Check sheet for the modelled part. Datum: model origin and axes. Units: mm. A direction names the side the tool comes from. Coordinates: 2 decimals unless noted, no trailing zeros. Write each loop counter-clockwise with the first axis right and the second up, starting at its lowest first coordinate (ties: lowest second). Pieces come first, ordered by that corner, then holes. Notation, with made-up numbers: (19.25, 49) - (30.25, 49) arc R15 ccw to (30.25, 76) - close; hole circle Ø11 at (-18, -28). An arc over 180 degrees is marked (long way). Use one line per item in the form item = value. Start each with the question number.
1. Tool access check on faces 1 (the face through (6, -2, -7)), 2 (the face through (3.436, 13.438, 8.76)), 3 (the face through (8.864, 13.438, 8.76)). Record the directions out of +Z, -Z, +X, -X, +Y, -Y that give a thin tool (end or side, any length) a straight path to the whole face; none if there is none.
2. Go/stop test with flat-tipped pins: pin 1 Ø6 at (x, z) = (8, -16) entering from -Y; pin 2 Ø1 at (x, z) = (3, -0.5) entering from +Y; pin 3 Ø1.4 at (x, y) = (4, 24.5) entering from +Z. Record where each tip stops, or that it passes through.
3. Cross-section at C-C on z = 7. Record the boundary of the cut face in (x, y).
4. Cross-section at D-D on y = 16.5. Record the boundary of the cut face in (x, z), then the cut area to 3 significant figures.
5. Cross-section at B-B on y = 1.5. Record the boundary of the cut face in (x, z).
6. Cross-section at A-A on y = 12.3. Record the boundary of the cut face in (x, z).
7. Draft check along Z on faces 4 (the face through (6.2, 24.9, -4)), 5 (the face through (3, 27.3, -5)), 6 (the face through (6.1, 15.2, 2.2)). Enter one of: +Z half, -Z half, draft (parallel to the pull), parting line (faces both ways), or undercut.
8. Scan lines: line 1 along X through (y, z) = (26.2, -4.95); line 2 along Z through (x, y) = (10, 3.5); line 3 along Z through (x, y) = (8.75, -1.5). Record each from-to range of solid material in increasing order.
Autodesk Inventor part; units mm, degrees
ref_plane "YZ Plane" through (0, 0, 0) normal (1, 0, 0) x (0, 1, 0)
ref_plane "XZ Plane" through (0, 0, 0) normal (0, 1, 0) x (-1, 0, 0)
ref_plane "XY Plane" through (0, 0, 0) normal (0, 0, 1) x (1, 0, 0)
sketch "Sketch1" plane through (0, 0, 0) normal (0, 0, 1) x (1, 0, 0)
  line L0 (0, 0) -> (12.3, 0)
  line L1 (12.3, 0) -> (12.3, 22.6)
  line L2 (12.3, 22.6) -> (0, 22.6)
  line L3 (0, 22.6) -> (0, 0)
  line L4 (6.15, 22.6) -> (6.15, 0) construction
  arc A0 (3.3318, 11.6163) -> (8.9682, 11.6163) centre (6.15, 6.15) ccw
  arc A1 (8.9682, 11.6163) -> (3.3318, 11.6163) centre (6.15, 12.3) ccw
  dimension "d0" = 12.3
  dimension "d1" = 22.6
  dimension "d2" = 6.15
  dimension "d3" = 6.15
  dimension "d4" = 5.8
extrude "Extrusion1" add sketch "Sketch1" against normal blind 22.3
sketch "Sketch2" plane through (0, 0, 0) normal (0, 0, 1) x (1, 0, 0)
  line L0 (0, 0) -> (12.3, 0)
  line L1 (12.3, 0) -> (12.3, 22.6)
  line L2 (12.3, 22.6) -> (0, 22.6)
  line L3 (0, 22.6) -> (0, 0)
  line L4 (6.15, 22.6) -> (6.15, 0) construction
  arc A0 (3.3318, 11.6163) -> (8.9682, 11.6163) centre (6.15, 6.15) ccw
  arc A1 (8.9682, 11.6163) -> (3.3318, 11.6163) centre (6.15, 12.3) ccw
  dimension "d7" = 12.3
  dimension "d8" = 22.6
  dimension "d9" = 6.15
  dimension "d10" = 6.15
  dimension "d11" = 5.8
extrude "Extrusion2" add sketch "Sketch2" along normal blind 4.5 contours A0 A1
sketch "Sketch3" plane through (0, 22.6, 0) normal (0, 1, 0) x (1, 0, 0)
  line L0 (12.3, 0) -> (0, 0) construction
  line L1 (12.3, 0) -> (12.3, 22.3) construction
  line L2 (0, 0) -> (0, 22.3) construction
  line L3 (12.3, 4) -> (0, 4)
  line L4 (0, 4) -> (0, 6.5)
  line L5 (0, 6.5) -> (12.3, 6.5)
  line L6 (12.3, 6.5) -> (12.3, 4)
  dimension "d14" = 4
  dimension "d15" = 2.5
extrude "Extrusion3" add sketch "Sketch3" along normal blind 4.7
sketch "Sketch4" plane through (0, 0, -22.3) normal (0, -1, 0) x (1, 0, 0)
  line L0 (12.3, 15.3) -> (0, 15.3)
  line L1 (0, 15.3) -> (0, 17.8)
  line L2 (0, 17.8) -> (12.3, 17.8)
  line L3 (12.3, 17.8) -> (12.3, 15.3)
  line L4 (0, 22.3) -> (6.15, 22.3) construction
  line L5 (0, 22.3) -> (0, 0) construction
  line L6 (12.3, 0) -> (0, 0) construction
  line L7 (12.3, 22.3) -> (12.3, 0) construction
  line L8 (6.15, 22.3) -> (12.3, 22.3) construction
  dimension "d19" = 2.5
  dimension "d20" = 4.5
extrude "Extrusion4" add sketch "Sketch4" along normal blind 4.7
sketch "Sketch5" plane through (0, 22.6, -4) normal (0, 0, 1) x (1, 0, 0)
  line L0 (12.3, 0) -> (0, 0) construction
  line L1 (12.3, 0) -> (12.3, 4.7) construction
  line L2 (0, 4.7) -> (12.3, 4.7) construction
  line L3 (0, 0) -> (0, 4.7) construction
  line L4 (0, 4.7) -> (12.3, 4.7)
  line L5 (6.15, 4.7) -> (6.15, 0)
  circle A0 centre (6.15, 3.6) radius 1.1
  point P0 (0, -22.6)
  dimension "d23" = 1.1
extrude "Extrusion5" cut sketch "Sketch5" against normal blind 10
sketch "Sketch6" plane through (0, 0, -4.5) normal (0, 0, 1) x (1, 0, 0)
  line L0 (0, 0) -> (12.3, 0) construction
  line L1 (0, 0) -> (0, -4.7) construction
  line L2 (12.3, -4.7) -> (0, -4.7) construction
  line L3 (12.3, 0) -> (12.3, -4.7) construction
  line L4 (0, -4.7) -> (12.3, -4.7) construction
  line L5 (6.15, -4.7) -> (6.15, 0) construction
  line L6 (12.3, 0) -> (0, 0) construction
  circle A0 centre (6.15, -3.6) radius 1.1
  dimension "d26" = 1.1
extrude "Extrusion6" cut sketch "Sketch6" against normal blind 10
sketch "Sketch7" plane through (0, 0, 4.5) normal (0, 0, 1) x (1, 0, 0)
  arc A0 (3.3318, 11.6163) -> (8.9682, 11.6163) centre (6.15, 6.15) ccw
  arc A1 (8.9682, 11.6163) -> (3.3318, 11.6163) centre (6.15, 12.3) ccw
  circle A2 centre (6.15, 6.15) radius 3.5
  point P0 (0, 0)
  dimension "d29" = 7
extrude "Extrusion7" add sketch "Sketch7" along normal blind 5 contours A2
sketch "Sketch8" plane through (6.15, 6.15, 9.5) normal (0, 0, 1) x (1, 0, 0)
  circle A0 centre (0, 0) radius 3.5 construction
  line L0 (0, 0) -> (0, 13.1535)
  circle A1 centre (0, 0) radius 3.5 construction
  arc A2 (1.9885, 14.0145) -> (-1.9885, 14.0145) centre (0, 13.8) ccw
  line L1 (-3.5, 0) -> (-1.9885, 14.0145)
  line L2 (3.5, 0) -> (1.9885, 14.0145)
  line L3 (0, -12.2559) -> (0, 3.5)
  line L4 (0, 15.8) -> (0, 18.1002)
  line L5 (3.5, 0) -> (-3.5, 0)
  point P0 (-6.15, -6.15)
  point P1 (0, -3.5)
  dimension "d32" = 19.3
  dimension "d33" = 2
extrude "Extrusion8" add sketch "Sketch8" against normal blind 1.5
properties part number "Servo"
Final values:
q1.face_1 = -Z, +X, -X, -Y
q1.face_2 = +Z, -X, +Y
q1.face_3 = +Z, +X, +Y
q2.pin_1 = 0
q2.pin_2 = 22.6
q2.pin_3 = -4
q3.outline = circle Ø7 at (6.15, 6.15)
q4.outline = (0, -22.3) - (12.3, -22.3) - (12.3, 0) - (0, 0) - close; (3.77, 8) - (8.53, 8) - (8.53, 9.5) - (3.77, 9.5) - close
q4.area = 281 mm²
q5.outline = (0, -22.3) - (12.3, -22.3) - (12.3, 0) - (10.17, 0) - (10.17, 4.5) - (2.13, 4.5) - (2.13, 0) - (0, 0) - close
q6.outline = (0, -22.3) - (12.3, -22.3) - (12.3, 0) - (9.05, 0) - (9.05, 4.5) - (3.25, 4.5) - (3.25, 0) - (0, 0) - close; (3.31, 8) - (8.99, 8) - (8.99, 9.5) - (3.31, 9.5) - close
q7.face_4 = +Z half
q7.face_5 = draft
q7.face_6 = undercut
q8.line_1 = 0 to 5.05, 7.25 to 12.3
q8.line_2 = -22.3 to 4.5
q8.line_3 = -7 to -4.5
